Source: CAD feature listing. Evaluate the final solid. Frame: model axes, mm. Round coordinates to 2 decimals unless told otherwise and drop trailing zeros. Write each loop counter-clockwise with the first axis right and the second up, starting at its lowest first coordinate (ties: lowest second). Pieces come first, ordered by that corner, then holes.
```python
from build123d import *

# Parameters (mm, degrees)
F3_W     = 75
F3_H     = 75
F3_W_2   = 60
F3_H_2   = 60
F4_DEPTH = 5
F5_D     = 5.1
F0_D     = 7.3
F1_D     = 5.1
F7_D     = 4.2


with BuildPart() as f4:
    # F3 (on Top) → F4 (new body)
    with BuildSketch(Plane.XY):
        Rectangle(F3_W, F3_H)
        Rectangle(F3_W_2, F3_H_2, mode=Mode.SUBTRACT)
        Rectangle(F3_W_2, F3_H_2)
    extrude(amount=F4_DEPTH)

    # F5 (through all)
    with Locations(Plane(origin=(0, 0, 0), x_dir=(1, 0, 0), z_dir=(0, 0, -1))):
        with Locations((-30, 30), (30, 30)):
            Hole(F5_D / 2)

    # F0 (through all)
    with Locations(Plane(origin=(0, 0, 0), x_dir=(1, 0, 0), z_dir=(0, 0, -1))):
        with Locations((-30, -30), (30, -30)):
            Hole(F0_D / 2)

    # F1 (through all)
    with Locations(Plane.XY.offset(5)):
        with Locations((0, 0), (0, -20)):
            Hole(F1_D / 2)

    # F7 (through all)
    with Locations(Plane.XY.offset(5)):
        with Locations((25, 0), (-25, 0)):
            Hole(F7_D / 2)


solid = f4.part
```
Q1. Line query: line 1 (Y direction, x = 0, z = 3.45); line 2 (X direction, y = 30, z = 1.65); line 3 (Y direction, x = -30, z = 1.35). Output: solid intervals per line, ascending.
Q2. Section query A-A, the plane x = -25. Output: boundary loops of the cut face in (y, z).
Q3. Section query C-C, the plane y = 30. Output: boundary loops of the cut face in (x, z), and give its area (3 significant figures).
Q4. Section query D-D, the plane x = 30.5. Output: boundary loops of the cut face in (y, z), and give its area (3 significant figures).
Q5. Pin query (flat end, axial travel): P1, Ø6, axis at x = 30, y = 30, coming from the -Z side. Return the tip coordinate at first contact, or that it passes through.
Q6. Section query B-B, the plane z = 3.55. Give the number of separate pieces and of enclosed holes in the cut face, and give its area (3 significant figures).
Q7. Mould query, pull axis X, two halves, no side actions, for faces 1 (the face through (37.5, -1, 2)), 2 (the face through (-37.5, -1, 2)), 3 (the face through (-28.1, -31.7, 2.5)). Classes: pulls with the +X half, pulls with the -X half, needs draft (parallel to the pull), parting line crosses it, or undercut.
Filled in:
1. line 1: y = -37.5 to -22.55, -17.45 to -2.55, 2.55 to 37.5
1. line 2: x = -37.5 to -33.65, -26.35 to 26.35, 33.65 to 37.5
1. line 3: y = -37.5 to -32.55, -27.45 to 26.35, 33.65 to 37.5
2. outline: (-37.5, 0) - (-2.1, 0) - (-2.1, 5) - (-37.5, 5) - close; (2.1, 0) - (37.5, 0) - (37.5, 5) - (2.1, 5) - close
3. outline: (-37.5, 0) - (-33.65, 0) - (-33.65, 5) - (-37.5, 5) - close; (-26.35, 0) - (26.35, 0) - (26.35, 5) - (-26.35, 5) - close; (33.65, 0) - (37.5, 0) - (37.5, 5) - (33.65, 5) - close
3. area: 302 mm2
4. outline: (-37.5, 0) - (-32.5, 0) - (-32.5, 5) - (-37.5, 5) - close; (-27.5, 0) - (26.38, 0) - (26.38, 5) - (-27.5, 5) - close; (33.62, 0) - (37.5, 0) - (37.5, 5) - (33.62, 5) - close
4. area: 314 mm2
5. P1: passes through
6. separate pieces: 1
6. enclosed holes: 8
6. area: 5,430 mm2
7. face 1: pulls with the +X half
7. face 2: pulls with the -X half
7. face 3: undercut
